Design review of the part built by this model. Coordinates are the model's own, in mm. A direction names the side the tool comes from. Give positions to 0.01 mm unless a question says otherwise; leave off trailing zeros. Loops run counter-clockwise (first coordinate to the right, second up) from the corner with the lowest first, then second, coordinate; pieces in that order, holes last. Notation, with made-up numbers: (-16.75, -39.5) -> (28.25, -39.5) arc R10 ccw to (28.25, -28.5) -> close; hole circle Ø7 at (-22.5, 32). An arc over 180 degrees is marked (long way). Answer as CSV lines item,"result".
from build123d import *

# Parameters (mm, degrees)
F1_DEPTH  = 127
F2_DEPTH  = 127
F3_D      = 25.4
F0_W      = 76.2
F0_H      = 76.2
F4_DEPTH  = 76.2
F6_D      = 25.4
F9_W      = 50.8
F9_H      = 76.2
F10_DEPTH = 25.4


# Not quite as in the source:
# - a feature of the source that left no trace in its solid (it failed there, or was rolled back) is left out
# - a feature names something its author has since deleted; it is built from what else it names


with BuildPart() as f1:
    # F0 (on Front) → F1 (new body)
    with BuildSketch(Plane.XZ):
        with BuildLine():
            Line((0, 0), (120.65, 0))
            ThreePointArc((120.65, 0), (85.3124331502, 85.3124331502), (0, 120.65))
            Line((0, 120.65), (0, 44.45))
            Line((0, 44.45), (0, 0))
        make_face()
    extrude(amount=-F1_DEPTH)

    # F0 (on Front) → F2 (join)
    with BuildSketch(Plane.XZ):
        Polygon((0, 44.45), (0, 120.65), (-19.05, 120.65), (-19.05, 44.45), (-19.05, 0), (0, 0), align=None)
    extrude(amount=-F2_DEPTH)

    # F3 (through all)
    with Locations(Plane.XZ):
        with Locations((57.15, 44.45)):
            Hole(F3_D / 2)

    # F0 (on Front) → F4 (join)
    with BuildSketch(Plane.XZ):
        with Locations((-57.15, 82.55)):
            Rectangle(F0_W, F0_H)
    extrude(amount=-F4_DEPTH)

    # F6 (through all)
    with Locations(Plane(origin=(-95.25, 0, 0), x_dir=(0, -1, 0), z_dir=(-1, 0, 0))):
        with Locations((-38.1, 88.9)):
            Hole(F6_D / 2)

    # F9 (on face) → F10 (join)
    with BuildSketch(Plane(origin=(-19.05, 0, 0), x_dir=(0, -1, 0), z_dir=(-1, 0, 0))):
        with Locations((-101.6, 82.55)):
            Rectangle(F9_W, F9_H)
    extrude(amount=F10_DEPTH)


solid = f1.part
Q1. To check wall thickness, follow probe 1 along Y at (x, z) = (13.5, 88.9); probe 2 along Z at (x, y) = (-45, 38). State the ranges of each line that lie inside material, in increasing order. Write a range as from..to.
Filled sheet:
probe 1,"y = 0..25.4, 50.8..127"
probe 2,"z = 44.45..76.2, 101.6..120.65"
Q2. We need section C-C, the plane z = 82.5. State the section outline as (x, y) points.
Filled sheet:
outline,"(-95.25, 0) -> (88.04, 0) -> (88.04, 27.13) -> (-95.25, 27.13) -> close; (-95.25, 49.07) -> (88.04, 49.07) -> (88.04, 127) -> (-44.45, 127) -> (-44.45, 76.2) -> (-95.25, 76.2) -> close"
Q3. We need section B-B, the plane y = 89.5. State the section outline as (x, z) points.
Filled sheet:
outline,"(-44.45, 44.45) -> (-19.05, 44.45) -> (-19.05, 0) -> (120.65, 0) arc R120.65 ccw to (0, 120.65) -> (-44.45, 120.65) -> close; hole circle Ø25.4 at (57.15, 44.45)"
Q4. Clearance check with flat-ended pins moving along their axes: pin 1 Ø2 at (y, z) = (36.5, 56.5) entering from +X; pin 2 Ø23 at (x, y) = (-68, 65.5) entering from -Z; pin 3 Ø13.5 at (y, z) = (53, 13) entering from -X; pin 4 Ø15 at (y, z) = (38.1, 88.9) entering from -X. State where each tip first meets the part, or that it passes through.
Filled sheet:
pin 1,"stops at x = 107.13"
pin 2,"stops at z = 44.45"
pin 3,"stops at x = -19.05"
pin 4,"passes through"
Q5. The part is to be moulded in two halves that separate along X. For faces 4 (the cylindrical face through (45.418, 64.389, 39.586)), 5 (the flat face through (-70, 76.2, 83)), 6 (the cylindrical face through (86.245, 62.611, 84.369)), say which applies: pulls with the +X half, pulls with the -X half, needs draft (parallel to the pull), parting line crosses it, or undercut.
Filled sheet:
face 4,"undercut"
face 5,"needs draft"
face 6,"pulls with the +X half"
Q6. For faces 1 (the flat face through (50, 63, 0)), 2 (the flat face through (-44.45, 102, 83)), 3 (the flat face through (-19.05, 63, 23)), list the 3-axis set-ups (+Z, -Z, +X, -X, +Y, -Y) from which the entire face can be reached by the end or side of a thin tool; tool diameter is ignored.
Filled sheet:
face 1,"-Z, +X, -X, +Y, -Y"
face 2,"+Z, -Z, -X, +Y"
face 3,"-Z, -X, +Y, -Y"
Q7. We need section D-D, the plane x = -9. State the section outline as (y, z) points, and give its area (3 significant figures).
Filled sheet:
outline,"(0, 0) -> (127, 0) -> (127, 120.65) -> (0, 120.65) -> close; hole circle Ø25.4 at (38.1, 88.9)"
area,"14,800 mm^2"
Q8. We need section A-A, the plane x = 59. State the section outline as (y, z) points.
Filled sheet:
outline,"(0, 0) -> (127, 0) -> (127, 31.89) -> (0, 31.89) -> close; (0, 57.01) -> (127, 57.01) -> (127, 105.24) -> (0, 105.24) -> close; hole circle Ø25.4 at (38.1, 88.9)"
